Geometry: see drawing. Coordinates: mm, zero at the bounding-box minimum. Round coordinates to 2 decimals unless told otherwise and drop trailing zeros. Write each loop counter-clockwise with the first axis right and the second up, starting at its lowest first coordinate (ties: lowest second). Pieces come first, ordered by that corner, then holes. Notation, with made-up numbers: M 28,5 L 59,5 A20 cw 59,38 Z; hole C 62,25.5 d1. An arc over 180 degrees is marked long. Use a Markdown table: item, result.
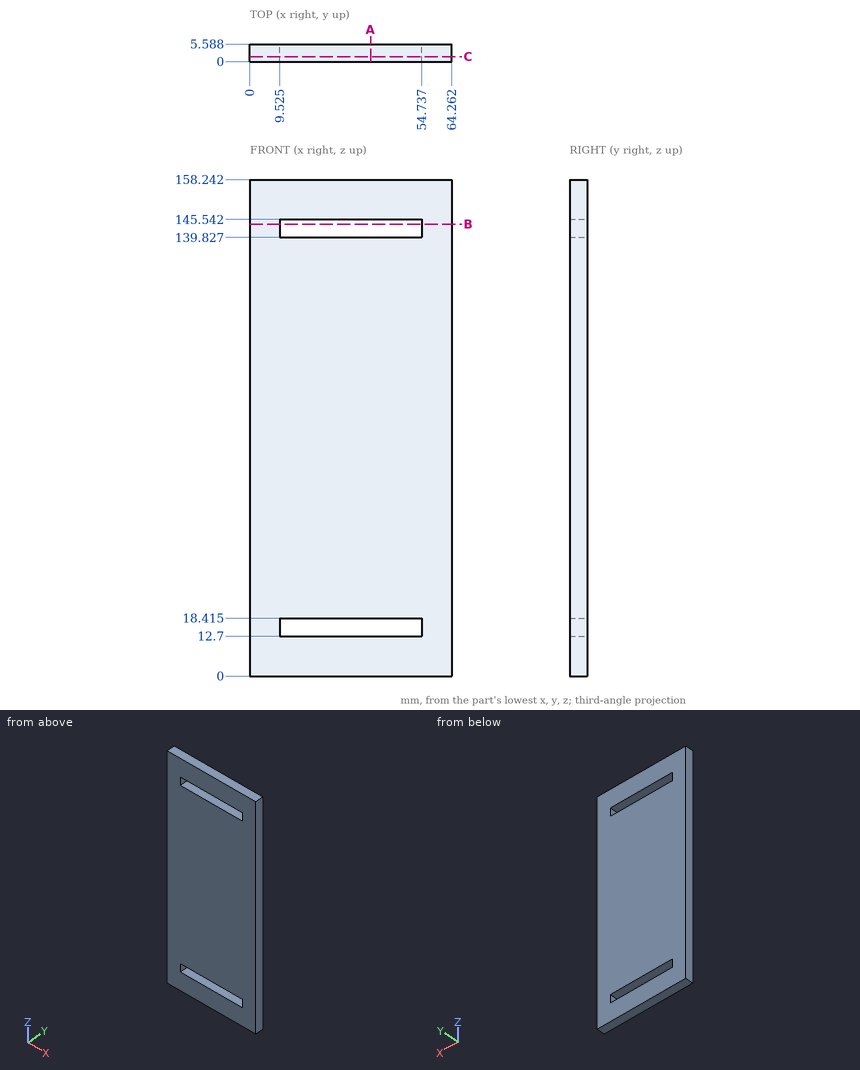
Q1. Line query: L1, parallel to Z at x = 17.5, y = 5.3 (3 decimals); L2, parallel to X at y = 2.3, z = 17.5 (3 decimals). Output: solid intervals per line, ascending.
Results are:
| item | result |
|---|---|
| L1 | 0 to 12.7, 18.415 to 139.827, 145.542 to 158.242 |
| L2 | 0 to 9.525, 54.737 to 64.262 |
Q2. Section B-B on z = 144. Return loops of the section in (x, y) (3 decimals).
Results are:
| item | result |
|---|---|
| outline | M 0,0 L 9.525,0 L 9.525,5.588 L 0,5.588 Z; M 54.737,0 L 64.262,0 L 64.262,5.588 L 54.737,5.588 Z |
Q3. Section A-A on x = 38.5. Return loops of the section in (y, z) (3 decimals).
Results are:
| item | result |
|---|---|
| outline | M 0,0 L 5.588,0 L 5.588,12.7 L 0,12.7 Z; M 0,18.415 L 5.588,18.415 L 5.588,139.827 L 0,139.827 Z; M 0,145.542 L 5.588,145.542 L 5.588,158.242 L 0,158.242 Z |
Q4. Section C-C on y = 1.6. Return loops of the section in (x, z) (3 decimals), plus the area to 3 significant figures.
Results are:
| item | result |
|---|---|
| outline | M 0,0 L 64.262,0 L 64.262,158.242 L 0,158.242 Z; hole M 9.525,12.7 L 54.737,12.7 L 54.737,18.415 L 9.525,18.415 Z; hole M 9.525,139.827 L 54.737,139.827 L 54.737,145.542 L 9.525,145.542 Z |
| area | 9,650 mm^2 |
